from build123d import *

# Parameters (mm, degrees)
SKETCH1_W           = 139.7
SKETCH1_H           = 6.35
BOSS_EXTRUDE1_DEPTH = 44.45
FILLET1_R           = 6.35
SKETCH4_R           = 3.96875
CUT_EXTRUDE2_DEPTH  = 254
SKETCH6_R           = 7.332348418
CUT_EXTRUDE4_DEPTH  = 3.81


with BuildPart() as part:
    # Sketch1 → Boss-Extrude1 (new body)
    with BuildSketch(Plane(origin=(0, 0, 0), x_dir=(1, 0, 0), z_dir=(0, 1, 0))):
        with Locations((69.85, 3.175)):
            Rectangle(SKETCH1_W, SKETCH1_H)
    extrude(amount=BOSS_EXTRUDE1_DEPTH)

    # Fillet1
    fillet1_edges = [part.edges().sort_by_distance(p)[0] for p in [
        (0, 22.225, -6.35),
    ]]
    fillet(fillet1_edges, radius=FILLET1_R - 0.0001)  # a hair under: the kernel refuses the full size

    # Sketch4 → Cut-Extrude2 (cut)
    with BuildSketch(Plane(origin=(69.948790088, 1.415162488, 139.7), x_dir=(1, 0, 0), z_dir=(0, 0, 1))):
        with Locations((-54.708790088, 20.809837512)):
            Circle(SKETCH4_R)
    extrude(amount=-CUT_EXTRUDE2_DEPTH, mode=Mode.SUBTRACT)

    # Sketch6 → Cut-Extrude4 (cut)
    with BuildSketch(Plane(origin=(0, 0, -6.35), x_dir=(-1, 0, 0), z_dir=(0, 0, -1))):
        with Locations((-15.24, 22.225)):
            Circle(SKETCH6_R)
    extrude(amount=-CUT_EXTRUDE4_DEPTH, mode=Mode.SUBTRACT)


solid = part.part
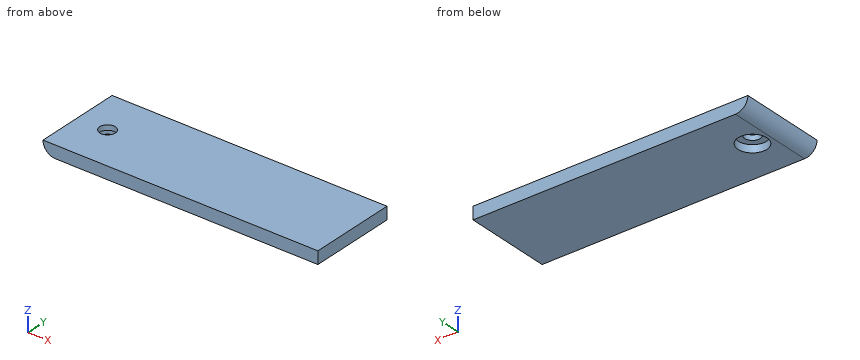
The listing builds one solid part. Answer for the finished solid, in the listing's coordinates (mm). Give positions to 0.01 mm unless a question says otherwise; leave off trailing zeros. Loops run counter-clockwise (first coordinate to the right, second up) from the corner with the lowest first, then second, coordinate; pieces in that order, holes last. Notation, with made-up numbers: (64, 76) - (82, 76) arc R16 ccw to (82, 106) - close; hole circle Ø8 at (27, 53.5). An arc over 180 degrees is marked (long way). Answer as a JSON object with one key per item and string values.
1. Find the intervals of material crossed by L1, parallel to Y at x = 15.24, z = -1.45; L2, parallel to Y at x = 15.24, z = -4.65; L3, parallel to X at y = 24, z = -5.5, in increasing order. Write a range as [from, to].
Determined:
{"L1": "[0, 18.26], [26.19, 44.45]", "L2": "[0, 14.89], [29.56, 44.45]", "L3": "[3.18, 8.13], [22.35, 139.7]"}
2. A cutting plane is placed at A-A (x = 15.24). Write down the section's boundary in (y, z).
Determined:
{"outline": "(0, -6.35) - (14.89, -6.35) - (14.89, -2.54) - (18.26, -2.54) - (18.26, 0) - (0, 0) - close; (26.19, -2.54) - (29.56, -2.54) - (29.56, -6.35) - (44.45, -6.35) - (44.45, 0) - (26.19, 0) - close"}
3. Flat-ended cylindrical pins translate along their axes: pin 1 Ø3 at (y, z) = (29.5, -4.5) entering from -X; pin 2 Ø7 at (x, y) = (15.24, 22.225) entering from -Z; pin 3 Ø2 at (y, z) = (17, -5) entering from -X; pin 4 Ø11.5 at (x, y) = (13, 20.5) entering from -Z. Find the tip coordinate at first contact, or state that the pin passes through.
Determined:
{"pin 1": "x = 0.75", "pin 2": "through", "pin 3": "x = 1.42", "pin 4": "z = -6.35"}
